from build123d import *

# Parameters (mm, degrees)
F2_R     = 1.4990506736
F3_DEPTH = 48.2092


with BuildPart() as f1:
    # F0 (on Front) → F1 (revolve)
    with BuildSketch(Plane.XZ):
        Polygon((6.8602792752, 1.8190295668), (11.4510266601, 1.8190295668), (6.8602792752, 3.0710518752), align=None)
        Polygon((-18.2348843664, 1.5875), (-18.2348843664, 0), (16.4666048384, 0), (16.4666048384, 1.8016344952), (11.8439664964, 3.0623543394), (11.8439664964, 1.8190295668), (11.4510266601, 1.8190295668), (6.8602792752, 1.8190295668), (6.499230396, 1.8190295668), (1.876592054, 1.8190295668), (1.0361127788, 1.8190295668), (1.0361127788, 4.2804344557), (0, 4.2804344557), (0, 1.5875), align=None)
        Polygon((1.876592054, 3.079749411), (1.876592054, 1.8190295668), (6.499230396, 1.8190295668), align=None)
    revolve(axis=Axis((-0.884139764, 0, 0), (1, 0, 0)))

    # F2 (on face) → F3 (cut)
    with BuildSketch(Plane.YZ.offset(16.4666048384)):
        Circle(F2_R)
    extrude(amount=-F3_DEPTH, mode=Mode.SUBTRACT)


solid = f1.part
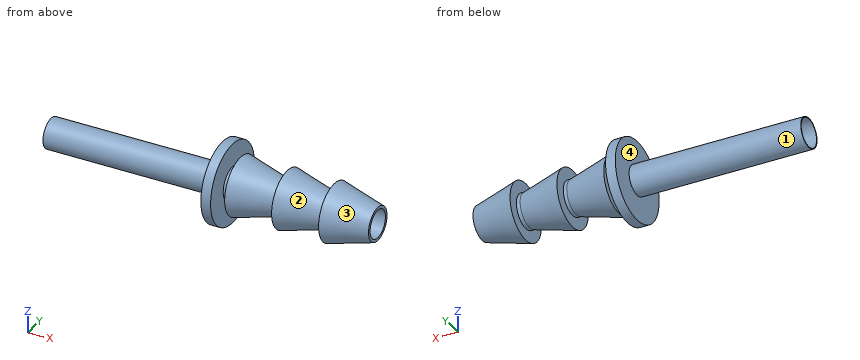
CAD build for the part. Positions are in the model's coordinates, mm. Face numbers are marked on the shaded views. Coordinates: 2 decimals unless noted, no trailing zeros. Write each loop counter-clockwise with the first axis right and the second up, starting at its lowest first coordinate (ties: lowest second). Pieces come first, ordered by that corner, then holes. Notation, with made-up numbers: (60, 46) - (82, 46) arc R17 ccw to (82, 60) - close; hole circle Ø9 at (-19.5, 12). An arc over 180 degrees is marked (long way). Use a Markdown table: item, result. Add a question column.
Item 1: Mould opens along X. For the marked faces 1, 2, 3 and 4 say: pulls with the +X half, pulls with the -X half, needs draft (parallel to the pull), parting line crosses it, or undercut.
Item 2: Drill centre lines: L1, parallel to X at y = 3, z = 3; L2, parallel to Y at x = 15, z = 1; L3, parallel to X at y = 0.75, z = -1.5. Where is each one in solid material? Low to high. Write a range as from..to.
Item 3: Flat gauge pins, fed straight in: pin 1 (4 mm diameter, centred on x = 5, y = -1, fed in from +Z); pin 2 (5 mm diameter, centred on y = 0, z = 0, fed in from +X); pin 3 (3 mm diameter, centred on x = 5.5, z = -0.5, fed in from -Y); pin 4 (4 mm diameter, centred on x = 11, y = -2.5, fed in from +Z). Where does each tip first touch, or does it go through?
Item 4: Band-saw the part on C-C, the plane x = -3.5. Give the cut face in (y, z) (1 decimal).
Item 5: Band-saw the part on D-D, the plane y = 2.5. Give the number of separate pieces and of enclosed holes in the cut face, and give its area (3 significant figures).
Numbers:
| question | item | result |
|---|---|---|
| 1 | face 1 | needs draft |
| 1 | face 2 | undercut |
| 1 | face 3 | pulls with the +X half |
| 1 | face 4 | pulls with the -X half |
| 2 | L1 | 0..1.04 |
| 2 | L2 | -1.96..-1.12, 1.12..1.96 |
| 2 | L3 | 0..16.47 |
| 3 | pin 1 | z = 3.06 |
| 3 | pin 2 | x = 16.47 |
| 3 | pin 3 | y = -3.07 |
| 3 | pin 4 | z = 2.98 |
| 4 | outline | circle Ø3.2 at (0, 0); hole circle Ø3 at (0, 0) |
| 5 | separate pieces | 4 |
| 5 | enclosed holes | 0 |
| 5 | area | 21.8 mm2 |
